Model file for the job. Use its own axes, mm. A direction names the side the tool comes from. Give positions to 0.01 mm unless a question says otherwise; leave off trailing zeros. Loops run counter-clockwise (first coordinate to the right, second up) from the corner with the lowest first, then second, coordinate; pieces in that order, holes last. Notation, with made-up numbers: M 85.5,10.25 L 96.5,10.25 A28 cw 96.5,49.25 Z; hole C -15.75,44 d11. An arc over 180 degrees is marked long. Answer in a Markdown table with one row per item.
```python
from build123d import *

# Parameters (mm, degrees)
ESQUISSE1_W             = 20
ESQUISSE1_H             = 20
ESQUISSE2_W             = 40
ESQUISSE2_H             = 40
ENL_V_MAT_EXTRU_1_DEPTH = 536.933764564


with BuildPart() as part:
    # Esquisse1 → Révolution1 (revolve)
    with BuildSketch(Plane.XY, mode=Mode.PRIVATE) as r_volution1_sk:
        Polygon((0, 0), (0, 290), (20, 290), (20, 150), (305, 150), (305, 290), (325, 290), (325, 0), align=None)
        with Locations((335, 280)):
            Rectangle(ESQUISSE1_W, ESQUISSE1_H)
        with Locations((-10, 280)):
            Rectangle(ESQUISSE1_W, ESQUISSE1_H)
    revolve(r_volution1_sk.sketch.rotate(Axis((0, 0, 0), (1, 0, 0)), 90), axis=Axis((0, 0, 0), (1, 0, 0)))

    # Esquisse2 → Enlèv. mat.-Extru.1 (cut, through all)
    with BuildSketch(Plane.ZY):
        Rectangle(ESQUISSE2_W, ESQUISSE2_H)
    extrude(amount=-ENL_V_MAT_EXTRU_1_DEPTH, mode=Mode.SUBTRACT)


solid = part.part
```
(1) Wall check: L1, parallel to X at y = -125.5, z = 145.5; L2, parallel to Y at x = -4, z = 0; L3, parallel to X at y = 262, z = 115.5. Give the ranges that are in metal, low to high.
Established:
| item | result |
|---|---|
| L1 | x = 0 to 20, 305 to 325 |
| L2 | y = -290 to -270, 270 to 290 |
| L3 | x = -20 to 20, 305 to 345 |
(2) Saw through at A-A, the plane y = 0. Give the cut face in (x, z).
Established:
| item | result |
|---|---|
| outline | M -20,-290 L 20,-290 L 20,-150 L 305,-150 L 305,-290 L 345,-290 L 345,-270 L 325,-270 L 325,-20 L 0,-20 L 0,-270 L -20,-270 Z; M -20,270 L 0,270 L 0,20 L 325,20 L 325,270 L 345,270 L 345,290 L 305,290 L 305,150 L 20,150 L 20,290 L -20,290 Z |
(3) Mould opens along X. For faces 1 (the cylindrical face through (-0.28, 257.28, 133.82)), 2 (the flat face through (345, 192, -192)), 3 (the flat face through (20, 125, 125)), 4 (the flat face through (-20, 192, -192)) say: pulls with the +X half, pulls with the -X half, needs draft (parallel to the pull), parting line crosses it, or undercut.
Established:
| item | result |
|---|---|
| face 1 | needs draft |
| face 2 | pulls with the +X half |
| face 3 | undercut |
| face 4 | pulls with the -X half |
(4) Which spindle directions (+Z, -Z, +X, -X, +Y, -Y) get a long thin tool onto all of the face, cutting with end or side? Do faces 5 (the cylindrical face through (-9.86, 164.291, -214.263)), 6 (the cylindrical face through (335.14, 164.291, -214.263)), 7 (the cylindrical face through (164.495, 133.076, 69.216)), 8 (the flat face through (160, -20, 0)). Say none if no direction does.
Established:
| item | result |
|---|---|
| face 5 | -X |
| face 6 | +X |
| face 7 | none |
| face 8 | +X, -X |
(5) Saw through at D-D, the plane y = 232. Give the cut face in (x, z), and give its area (3 significant figures).
Established:
| item | result |
|---|---|
| outline | M -20,-174 L 20,-174 L 20,174 L -20,174 L -20,138.12 L 0,138.12 L 0,-138.12 L -20,-138.12 Z; M 305,-174 L 345,-174 L 345,-138.12 L 325,-138.12 L 325,138.12 L 345,138.12 L 345,174 L 305,174 Z |
| area | 16,800 mm2 |
(6) Flat gauge pins, fed straight in: P1, Ø1, axis at y = 133.5, z = 206, coming from the +X side; P2, Ø2, axis at y = 70, z = -14.5, coming from the -X side; P3, Ø6, axis at x = 152, z = 17.5, coming from the +Y side. Where does each tip first touch, or does it go through?
Established:
| item | result |
|---|---|
| P1 | stops at x = 325 |
| P2 | stops at x = 0 |
| P3 | stops at y = 149.3 |
(7) Saw through at C-C, the plane x = 208. Give the cut face in (y, z), and give its area (3 significant figures).
Established:
| item | result |
|---|---|
| outline | C 0,0 d300; hole M -20,-20 L 20,-20 L 20,20 L -20,20 Z |
| area | 69,100 mm2 |
